```python
from build123d import *

# Parameters (mm, degrees)
SKETCH_1_R         = 1.65
SKETCH_1_R_2       = 5.5
EXTRUDE_4604_DEPTH = 2
FILLET_1_R         = 2


with BuildPart() as part:
    # Эскиз1 → Extrude 4604 (new body)
    with BuildSketch(Plane(origin=(0, 0, 0), x_dir=(1, 0, 0), z_dir=(0, 1, 0))):
        with BuildLine():
            Line((-11.508257905, -3.4), (-29.714194139, -8.778762251))
            ThreePointArc((-29.714194139, -8.778762251), (-45.087395339, -25.73505383), (-37.075043377, -47.1745817))
            ThreePointArc((-37.075043377, -47.1745817), (-17.087040134, -57.515502775), (5.304800773, -59.765032325))
            ThreePointArc((5.304800773, -59.765032325), (22.603580264, -48.512957528), (22.97025793, -27.879913482))
            ThreePointArc((22.97025793, -27.879913482), (21.591479888, -13.237630517), (30.59852352, -1.611339436))
            ThreePointArc((30.59852352, -1.611339436), (49.34717261, 15.870005048), (59.088465181, 39.58110934))
            ThreePointArc((59.088465181, 39.58110934), (54.221507729, 46.531844924), (47.270772145, 41.664887472))
            ThreePointArc((47.270772145, 41.664887472), (35.068418794, 17.224917951), (11.508257905, 3.4))
            ThreePointArc((11.508257905, 3.4), (-3.4, 11.508257905), (-11.508257905, -3.4))
        make_face()
        with Locations(Location((-1.510792129, -55.97961689, 0), (0, 0, 90))):
            Circle(SKETCH_1_R, mode=Mode.SUBTRACT)
        with Locations(Location((-29.298192809, -47.724374256, 0), (0, 0, 270))):
            Circle(SKETCH_1_R, mode=Mode.SUBTRACT)
        with Locations(Location((0, 0, 0), (0, 0, 270))):
            Circle(SKETCH_1_R_2, mode=Mode.SUBTRACT)
        with Locations(Location((8.627325416, -2.56305602, 0), (0, 0, 270))):
            Circle(SKETCH_1_R, mode=Mode.SUBTRACT)
        with Locations(Location((-6.533334333, -6.189954967, 0), (0, 0, 270))):
            Circle(SKETCH_1_R, mode=Mode.SUBTRACT)
        with Locations(Location((-2.093991083, 8.753010987, 0), (0, 0, 270))):
            Circle(SKETCH_1_R, mode=Mode.SUBTRACT)
        with Locations(Location((53.179618663, 40.622998406, 0), (0, 0, 270))):
            Circle(SKETCH_1_R, mode=Mode.SUBTRACT)
        with Locations(Location((46.765371804, 23, 0), (0, 0, 270))):
            Circle(SKETCH_1_R, mode=Mode.SUBTRACT)
        with Locations(Location((34.710530923, 8.633600072, 0), (0, 0, 270))):
            Circle(SKETCH_1_R, mode=Mode.SUBTRACT)
        with BuildLine():
            Line((-19.493884775, -16.456951096), (7.346683187, -24.430903158))
            ThreePointArc((7.346683187, -24.430903158), (17.289589147, -39.25061121), (4.597494003, -51.796361348))
            ThreePointArc((4.597494003, -51.796361348), (-14.808768116, -49.846769072), (-32.13170426, -40.884637473))
            ThreePointArc((-32.13170426, -40.884637473), (-35.915324215, -23.444186054), (-19.493884775, -16.456951096))
        make_face(mode=Mode.SUBTRACT)
    extrude(amount=EXTRUDE_4604_DEPTH)

    # Скругление1
    fillet_1_edges = [part.edges().sort_by_distance(p)[0] for p in [
        (-11.508257905, 1, 3.4),
        (11.508257905, 1, -3.4),
    ]]
    fillet(fillet_1_edges, radius=FILLET_1_R)


solid = part.part
```
Work out the finished part from the listing and answer in its coordinate system (mm). A direction names the side the tool comes from. Round coordinates to 2 decimals unless told otherwise and drop trailing zeros. Loops run counter-clockwise (first coordinate to the right, second up) from the corner with the lowest first, then second, coordinate; pieces in that order, holes last. Notation, with made-up numbers: M 68.25,47.5 L 104.25,47.5 A7 cw 104.25,60.5 Z; hole C 33.5,81 d8. An arc over 180 degrees is marked long. One line per question, with ' | ' between items.
Q1. Each of these flat-tipped pins is pushed along its axis until it touches: pin 1 Ø3 at (x, z) = (-1.51, 55.98) entering from +Y; pin 2 Ø1 at (x, y) = (0, 1.5) entering from -Z; pin 3 Ø1 at (x, y) = (6.5, 1) entering from +Z. Where does it stop, or does it pass through?
Conclusion:
pin 1: passes through | pin 2: stops at z = -12 | pin 3: stops at z = 59.69
Q2. Find section C-C, the plane x = 38. Give the vertices of the cut face in (y, z), then the cut area to 3 significant figures.
Conclusion:
outline: M 0,-20.67 L 2,-20.67 L 2,-3.57 L 0,-3.57 Z | area: 34.2 mm2
Q3. Find section B-B, the plane z = -23. Give the vertices of the cut face in (x, y), then the cut area to 3 significant figures.
Conclusion:
outline: M 39.69,0 L 45.12,0 L 45.12,2 L 39.69,2 Z; M 48.42,0 L 53.58,0 L 53.58,2 L 48.42,2 Z | area: 21.2 mm2
Q4. Find section A-A, the plane z = 34. Give the vertices of the cut face in (x, y).
Conclusion:
outline: M -45.09,0 L -36.86,0 L -36.86,2 L -45.09,2 Z; M 16.82,0 L 25.02,0 L 25.02,2 L 16.82,2 Z
Q5. A tool of negligible diameter and unlimited length cuts with its end or side. For faces 1 (the cylindrical face through (35.943, 0.986, -18.187)), 2 (the cylindrical face through (17.314, 0.986, 38.981)), 3 (the cylindrical face through (21.534, 0.986, 13.44)), from which of +Z, -Z, +X, -X, +Y, -Y can it reach the whole face along a straight path? Write none if from no direction.
Conclusion:
face 1: -Z, +Y, -Y | face 2: +Y, -Y | face 3: +X, +Y, -Y
Q6. Find section D-D, the plane y = 1.35. State how many separate pieces and enclosed holes the cut face has, then the cut area to 3 significant figures.
Conclusion:
separate pieces: 1 | enclosed holes: 10 | area: 2,750 mm2
Q7. The mould has two halves that part along X. Classify faces 4 (the cylindrical face through (-36.04, 0.99, 23.69)), 5 (the flat face through (7, 0, 10)), 6 (the cylindrical face through (49.14, 0.99, -15.57)): +X half, -X half, draft (parallel to the pull), parting line (faces both ways), or undercut.
Conclusion:
face 4: undercut | face 5: draft | face 6: +X half
Q8. Consider line 1 along Z through (x, y) = (-7, 0.65); line 2 along X through (y, z) = (1.85, 48) (3 decimals); line 3 along X through (y, z) = (0.8, -23). Determine where each line is inside the solid, lowest interval first. Write a range as from..to.
Conclusion:
line 1: z = -9.75..4.61, 7.77..20.17, 51.53..59.59 | line 2: x = -36..-30.925, -27.671..-20, 13.003..22.879 | line 3: x = 39.69..45.12, 48.42..53.58
